```python
from build123d import *

# Parameters (mm, degrees)
SKETCH1_R           = 3.7592
SKETCH1_R_2         = 1.397
BOSS_EXTRUDE1_DEPTH = 1.5875
CUT_EXTRUDE1_DEPTH  = 83.87509024
FILLET1_R           = 5.08
FILLET2_R           = 5.08
CUT_EXTRUDE2_REACH  = 82.757
BOSS_EXTRUDE2_DEPTH = 1.5875
FILLET3_R           = 5.08
CUT_EXTRUDE3_REACH  = 82.757
FILLET4_R           = 0.762


with BuildPart() as part:
    # Sketch1 → Boss-Extrude1 (new body)
    with BuildSketch(Plane.XY):
        Polygon((59.817595463, 0.441306322), (64.845697084, 21.910029909), (33.226760771, 51.582904103), (12.120249948, 45.203006047), (2.232255249, 2.983766862), (18.31066445, -12.105058669), align=None)
        with Locations((31.758870494, 18.335992429)):
            Circle(SKETCH1_R, mode=Mode.SUBTRACT)
        with Locations((13.143651596, -1.500084688)):
            Circle(SKETCH1_R_2, mode=Mode.SUBTRACT)
        with Locations((58.245026637, 12.132778525)):
            Circle(SKETCH1_R_2, mode=Mode.SUBTRACT)
        with Locations((23.887933249, 44.37528345)):
            Circle(SKETCH1_R_2, mode=Mode.SUBTRACT)
    extrude(amount=BOSS_EXTRUDE1_DEPTH)

    # Sketch2 → Cut-Extrude1 (cut, through all)
    with BuildSketch(Plane(origin=(0, 0, 0), x_dir=(-1, 0, 0), z_dir=(0, 0, -1))):
        Polygon((-33.226760771, 51.582904103), (-64.845697084, 21.910029909), (-34.366094464, 21.114208254), align=None)
        Polygon((-28.049253027, 19.204806708), (-2.232255249, 2.983766862), (-12.120249948, 45.203006047), align=None)
        Polygon((-32.861263991, 14.688962325), (-18.31066445, -12.105058669), (-59.817595463, 0.441306322), align=None)
    extrude(amount=-CUT_EXTRUDE1_DEPTH, mode=Mode.SUBTRACT)

    # Fillet1
    fillet1_edges = [part.edges().sort_by_distance(p)[0] for p in [
        (34.366094464, 21.114208254, 0.79375),
        (28.049253027, 19.204806708, 0.79375),
        (32.861263991, 14.688962325, 0.79375),
    ]]
    fillet(fillet1_edges, radius=FILLET1_R)

    # Fillet2
    fillet2_edges = [part.edges().sort_by_distance(p)[0] for p in [
        (18.31066445, -12.105058669, 0.79375),
        (2.232255249, 2.983766862, 0.79375),
        (12.120249948, 45.203006047, 0.79375),
        (33.226760771, 51.582904103, 0.79375),
        (64.845697084, 21.910029909, 0.79375),
        (59.817595463, 0.441306322, 0.79375),
    ]]
    fillet(fillet2_edges, radius=FILLET2_R)

    # Sketch3 → Cut-Extrude2 (cut, up to next)
    with BuildSketch(Plane(origin=(0, 0, 0), x_dir=(-1, 0, 0), z_dir=(0, 0, -1)), mode=Mode.PRIVATE) as cut_extrude2_sk1:
        with BuildLine():
            ThreePointArc((-27.999670494, 18.335992429), (-28.12209579, 17.384438756), (-28.481397666, 16.494863291))
            Line((-28.481397666, 16.494863291), (-24.797711818, 17.357604232))
            ThreePointArc((-24.797711818, 17.357604232), (-26.039580674, 19.67548382), (-25.956130857, 22.303760854))
            Line((-25.956130857, 22.303760854), (-29.639816705, 21.441019913))
            ThreePointArc((-29.639816705, 21.441019913), (-28.434902109, 20.091788208), (-27.999670494, 18.335992429))
        make_face()
    cut_extrude2_tool1 = extrude(cut_extrude2_sk1.sketch, amount=-CUT_EXTRUDE2_REACH, mode=Mode.PRIVATE) & part.part
    add(cut_extrude2_tool1.solids().sort_by_distance((27.120451, 19.422338, 0))[0], mode=Mode.SUBTRACT)

    # Sketch4 → Boss-Extrude2 (add)
    with BuildSketch(Plane.XY.offset(1.5875)):
        Polygon((32.680495966, 18.941790424), (35.601454601, 18.257684693), (35.236598188, 16.699839988), (32.315639553, 17.383945719), align=None)
    extrude(amount=-BOSS_EXTRUDE2_DEPTH)

    # Fillet3
    fillet3_edges = [part.edges().sort_by_distance(p)[0] for p in [
        (25.956130857, 22.303760854, 0.79375),
        (24.797711818, 17.357604232, 0.79375),
    ]]
    fillet(fillet3_edges, radius=FILLET3_R)

    # Sketch5 → Cut-Extrude3 (cut, up to next)
    with BuildSketch(Plane.XY.offset(1.5875), mode=Mode.PRIVATE) as cut_extrude3_sk1:
        Polygon((30.303711078, 23.150072166), (30.303711078, 43.528414036), (19.015506314, 40.116310717), align=None)
    cut_extrude3_tool1 = extrude(cut_extrude3_sk1.sketch, amount=-CUT_EXTRUDE3_REACH, mode=Mode.PRIVATE) & part.part
    # Sketch5 → Cut-Extrude3 (cut, up to next)
    with BuildSketch(Plane.XY.offset(1.5875), mode=Mode.PRIVATE) as cut_extrude3_sk2:
        Polygon((36.65556555, 17.189157581), (54.303727297, 6.999986646), (56.992861524, 18.481910394), align=None)
    cut_extrude3_tool2 = extrude(cut_extrude3_sk2.sketch, amount=-CUT_EXTRUDE3_REACH, mode=Mode.PRIVATE) & part.part
    # Sketch5 → Cut-Extrude3 (cut, up to next)
    with BuildSketch(Plane.XY.offset(1.5875), mode=Mode.PRIVATE) as cut_extrude3_sk3:
        Polygon((28.317334854, 14.66874754), (10.669173107, 4.479576605), (19.268243644, -3.590243825), align=None)
    cut_extrude3_tool3 = extrude(cut_extrude3_sk3.sketch, amount=-CUT_EXTRUDE3_REACH, mode=Mode.PRIVATE) & part.part
    add(cut_extrude3_tool1.solids().sort_by_distance((26.540976, 35.598266, 1.5875))[0], mode=Mode.SUBTRACT)
    add(cut_extrude3_tool2.solids().sort_by_distance((49.317385, 14.223685, 1.5875))[0], mode=Mode.SUBTRACT)
    add(cut_extrude3_tool3.solids().sort_by_distance((19.418251, 5.186027, 1.5875))[0], mode=Mode.SUBTRACT)

    # Fillet4
    fillet4_edges = [part.edges().sort_by_distance(p)[0] for p in [
        (19.015506314, 40.116310717, 0.79375),
        (30.303711078, 43.528414036, 0.79375),
        (30.303711078, 23.150072166, 0.79375),
        (56.992861524, 18.481910394, 0.79375),
        (54.303727297, 6.999986646, 0.79375),
        (36.65556555, 17.189157581, 0.79375),
        (19.268243644, -3.590243825, 0.79375),
        (10.669173107, 4.479576605, 0.79375),
        (28.317334854, 14.66874754, 0.79375),
    ]]
    fillet(fillet4_edges, radius=FILLET4_R)


solid = part.part
```
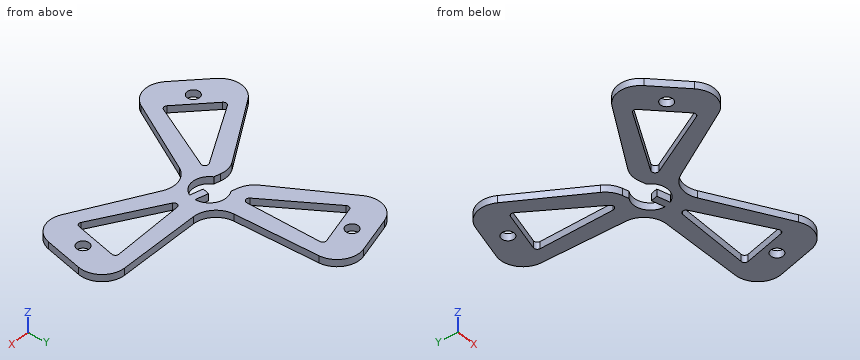
Geometry: final body of the model. Coordinates: model frame, mm. Round coordinates to 2 decimals unless told otherwise and drop trailing zeros. Order: outer loops, then holes, each group sorted by start corner. A loop starts at its lowest first (then second) coordinate and runs counter-clockwise, first axis right, second up. Notation, with made-up numbers: (55, -15) -> (74, -15) arc R11 ccw to (74, -7) -> close; hole circle Ø1 at (67, 51). An arc over 180 degrees is marked (long way). Use one line per item in the form item = value. Start each with the question number.
1. Cut plane B-B (y = 31.5). Return the cut outline in (x, z).
2. Line query: probe 1 along Y at (x, z) = (13, 0.95); probe 2 along X at (y, z) = (10.5, 0.25); probe 3 along X at (y, z) = (13, 0.45). Output: solid intervals per line, ascending.
3. Pin query (flat end, axial travel): pin 1 Ø2 at (x, y) = (23.89, 44.38) entering from +Z. Return the tip coordinate at first contact, or that it passes through.
4. Cut plane D-D (z = 0.5). Count the separate pieces of the cut face and the enclosed holes in it, then the cut area to 3 significant figures.
5. Cut plane A-A (x = 52.5). Return the cut outline in (y, z), then the cut area to 3 significant figures.
6. Cut plane C-C (x = 16.5). Return the cut outline in (y, z), then the cut area to 3 significant figures.
Solution:
q1.outline = (20.52, 0) -> (24.75, 0) -> (24.75, 1.59) -> (20.52, 1.59) -> close; (30.3, 0) -> (33.98, 0) -> (33.98, 1.59) -> (30.3, 1.59) -> close
q2.probe_1 = -7.12 to -2.89, -0.11 to 2.29, 5.83 to 9.75
q2.probe_2 = 14.19 to 21.1, 26.25 to 30.59, 40.79 to 48.24, 55.12 to 62.17
q2.probe_3 = 18.17 to 25.43, 27.23 to 43.91, 55.71 to 57.15, 59.34 to 62.76
q3.pin_1 = through
q4.separate_pieces = 1
q4.enclosed_holes = 6
q4.area = 831 mm^2
q5.outline = (4.31, 0) -> (8.04, 0) -> (8.04, 1.59) -> (4.31, 1.59) -> close; (18.2, 0) -> (21.59, 0) -> (21.59, 1.59) -> (18.2, 1.59) -> close
q5.area = 11.3 mm^2
q6.outline = (-8.95, 0) -> (-0.99, 0) -> (-0.99, 1.59) -> (-8.95, 1.59) -> close; (7.85, 0) -> (11.95, 0) -> (11.95, 1.59) -> (7.85, 1.59) -> close; (38.05, 0) -> (46.03, 0) -> (46.03, 1.59) -> (38.05, 1.59) -> close
q6.area = 31.8 mm^2
